Here's how the part is built. I have some questions about the finished solid (model axes, mm). A direction names the side the tool comes from. Coordinates: 2 decimals unless noted, no trailing zeros. Write each loop counter-clockwise with the first axis right and the second up, starting at its lowest first coordinate (ties: lowest second). Pieces come first, ordered by that corner, then holes. Notation, with made-up numbers: (-26.5, 72.25) -> (30.5, 72.25) arc R8 cw to (30.5, 76.25) -> close; hole circle Ø4 at (-27, -38.5). An arc over 180 degrees is marked (long way). Put each result on its own line as item: value.
```python
from build123d import *

# Parameters (mm, degrees)
SKETCH1_R           = 17.4
SKETCH1_R_2         = 1.75
SKETCH1_R_3         = 7.5
BOSS_EXTRUDE1_DEPTH = 4.5
CUT_EXTRUDE1_START  = -0.5
SKETCH2_R           = 9.2
CUT_EXTRUDE1_DEPTH  = 4
SKETCH3_R           = 15.25
SKETCH3_R_2         = 11.75
BOSS_EXTRUDE2_DEPTH = 1.5
CHAMFER1_SIZE       = 0.5
SKETCH4_R           = 17.9
SKETCH4_R_2         = 17.4
BOSS_EXTRUDE3_DEPTH = 2
SKETCH5_R           = 2.35
CUT_EXTRUDE2_DEPTH  = 4
CHAMFER3_SIZE       = 0.4


with BuildPart() as part:
    # Sketch1 → Boss-Extrude1 (new body, symmetric)
    with BuildSketch(Plane(origin=(0, 0, 0), x_dir=(1, 0, 0), z_dir=(0, 1, 0))):
        Circle(SKETCH1_R)
        with Locations((13.5, 0)):
            Circle(SKETCH1_R_2, mode=Mode.SUBTRACT)
        with Locations((6.75, -11.691342951)):
            Circle(SKETCH1_R_2, mode=Mode.SUBTRACT)
        with Locations((-6.75, -11.691342951)):
            Circle(SKETCH1_R_2, mode=Mode.SUBTRACT)
        with Locations((-13.5, 0)):
            Circle(SKETCH1_R_2, mode=Mode.SUBTRACT)
        with Locations((-6.75, 11.691342951)):
            Circle(SKETCH1_R_2, mode=Mode.SUBTRACT)
        with Locations((6.75, 11.691342951)):
            Circle(SKETCH1_R_2, mode=Mode.SUBTRACT)
        Circle(SKETCH1_R_3, mode=Mode.SUBTRACT)
    extrude(amount=BOSS_EXTRUDE1_DEPTH, both=True)

    # Sketch2 → Cut-Extrude1 (cut)
    with BuildSketch(Plane(origin=(0, 0, 0), x_dir=(1, 0, 0), z_dir=(0, 1, 0)).offset(CUT_EXTRUDE1_START)):
        Circle(SKETCH2_R)
    extrude(amount=CUT_EXTRUDE1_DEPTH, mode=Mode.SUBTRACT)

    # Sketch3 → Boss-Extrude2 (add)
    with BuildSketch(Plane.XZ.offset(4.5)):
        Circle(SKETCH3_R)
        Circle(SKETCH3_R_2, mode=Mode.SUBTRACT)
    extrude(amount=-BOSS_EXTRUDE2_DEPTH)

    # Chamfer1
    chamfer1_edges = [part.edges().sort_by_distance(p)[0] for p in [
        (-7.5, -4.5, 0),
        (-7.5, 4.5, 0),
    ]]
    chamfer(chamfer1_edges, length=CHAMFER1_SIZE)

    # Sketch4 → Boss-Extrude3 (add)
    with BuildSketch(Plane(origin=(0, 4.5, 0), x_dir=(1, 0, 0), z_dir=(0, 1, 0))):
        Circle(SKETCH4_R)
        Circle(SKETCH4_R_2, mode=Mode.SUBTRACT)
    extrude(amount=-BOSS_EXTRUDE3_DEPTH)

    # Sketch5 → Cut-Extrude2 (cut)
    with BuildSketch(Plane(origin=(0, -4.5, 0), x_dir=(-1, 0, 0), z_dir=(0, -1, 0))):
        with Locations((-9.742785793, -5.625)):
            Circle(SKETCH5_R)
        with Locations((-9.742785793, 5.625)):
            Circle(SKETCH5_R)
        with Locations((0, 11.25)):
            Circle(SKETCH5_R)
        with Locations((9.742785793, 5.625)):
            Circle(SKETCH5_R)
        with Locations((9.742785793, -5.625)):
            Circle(SKETCH5_R)
        with Locations((0, -11.25)):
            Circle(SKETCH5_R)
    extrude(amount=-CUT_EXTRUDE2_DEPTH, mode=Mode.SUBTRACT)

    # Chamfer3
    chamfer3_edges = [part.edges().sort_by_distance(p)[0] for p in [
        (-17.9, 4.5, 0),
        (-17.4, -4.5, 0),
    ]]
    chamfer(chamfer3_edges, length=CHAMFER3_SIZE)


solid = part.part
```
Item 1: If we mould it in two halves opening along X, with no side actions, what happens to faces 5 (the flat face through (8, 4.5, 4)), 6 (the flat face through (0, -0.5, 11))? For each: released by +X, released by -X, zero draft, split by the parting line, or undercut.
Output:
face 5: zero draft
face 6: undercut
Item 2: For P1, Ø2, axis at x = 11, y = 0, coming from the -Z side; P2, Ø2, axis at x = 11.5, y = 0.5, coming from the +Z side; P3, Ø1, axis at x = 13, z = 0.5, coming from the +Y side, each with a flat end and sliding along its axis, tell me the tip position at first contact or that it passes through.
Output:
P1: stops at z = -14.24
P2: stops at z = 13.87
P3: stops at y = -3
Item 3: Please list where these lines run through material, in increasing order: line 1 along X through (y, z) = (2.4, 0); line 2 along Z through (x, y) = (0, 1); line 3 along X through (y, z) = (3.25, -13). Write a range as from..to.
Output:
line 1: x = -17.4..-15.25, -11.75..-9.2, 9.2..11.75, 15.25..17.4
line 2: z = -17.4..-9.2, 9.2..17.4
line 3: x = -12.3..-7.91, -5.59..5.59, 7.91..12.3
Item 4: Imagine slicing it at A-A on y = 0. Write out the boundary of the cut face in (x, z), then the cut area to 3 significant figures.
Output:
outline: circle Ø34.8 at (0, 0); hole circle Ø3.5 at (-13.5, 0); hole circle Ø18.4 at (0, 0); hole circle Ø3.5 at (-6.75, -11.69); hole circle Ø3.5 at (-6.75, 11.69); hole circle Ø3.5 at (6.75, -11.69); hole circle Ø3.5 at (6.75, 11.69); hole circle Ø3.5 at (13.5, 0)
area: 628 mm²
Item 5: Which directions (+Z, -Z, +X, -X, +Y, -Y) give clear straight access to the entire face, cutting with the end or side of a thin tool? Please do faces 1 (the cylindrical face through (-7.3, 1.5, 5.6)), 2 (the cylindrical face through (0.509, -2.528, -8.956)), 3 (the flat face through (-7, -3, -12)), 4 (the flat face through (-4, -4.5, 7.3)).
Output:
face 1: none
face 2: -Y
face 3: +Y
face 4: +Z, -Z, +X, -X, -Y
